Source: CAD feature listing. Evaluate the final solid. Frame: model axes, mm. A direction names the side the tool comes from. Round coordinates to 2 decimals unless told otherwise and drop trailing zeros. Order: outer loops, then holes, each group sorted by start corner. A loop starts at its lowest first (then second) coordinate and runs counter-clockwise, first axis right, second up.
```python
from build123d import *

# Parameters (mm, degrees)
SALIENTE_EXTRUIR1_DEPTH                              = 6.35
REFRENTADO_PARA_TORNILLO_CON_CABEZA_HUEC_D           = 6.7564
REFRENTADO_PARA_TORNILLO_CON_CABEZA_HUEC_CBORE_D     = 11.1125
REFRENTADO_PARA_TORNILLO_CON_CABEZA_HUEC_CBORE_DEPTH = 6.35


with BuildPart() as part:
    # Croquis1 → Saliente-Extruir1 (new, symmetric)
    with BuildSketch(Plane.XY):
        with BuildLine():
            Line((43.5, 63.5), (-43.5, 63.5))
            ThreePointArc((-43.5, 63.5), (-57.642135624, 57.642135624), (-63.5, 43.5))
            Line((-63.5, 43.5), (-63.5, -63.5))
            Line((-63.5, -63.5), (63.5, -63.5))
            Line((63.5, -63.5), (63.5, 43.5))
            ThreePointArc((63.5, 43.5), (57.642135624, 57.642135624), (43.5, 63.5))
        make_face()
    extrude(amount=SALIENTE_EXTRUIR1_DEPTH, both=True)

    # Refrentado para tornillo con cabeza hueca de 1/41 (through all)
    with Locations(Plane(origin=(0, 0, -6.35), x_dir=(-1, 0, 0), z_dir=(0, 0, -1))):
        with Locations((43.85, 34.1), (43.85, 2.1), (-43.85, 2.1), (-43.85, 34.1)):
            CounterBoreHole(REFRENTADO_PARA_TORNILLO_CON_CABEZA_HUEC_D / 2, REFRENTADO_PARA_TORNILLO_CON_CABEZA_HUEC_CBORE_D / 2, REFRENTADO_PARA_TORNILLO_CON_CABEZA_HUEC_CBORE_DEPTH)


solid = part.part
```
1. Line query: line 1 along Y through (x, z) = (-43.85, -3); line 2 along Y through (x, z) = (43.85, 4.5); line 3 along X through (y, z) = (7, -1.5). Output: solid intervals per line, ascending.
2. Pull-direction query (Y, two-part tool) for faces 1 (the face through (-46.531, 32.044, 3.219)), 2 (the face through (-63.5, -9, 0)), 3 (the face through (-57.486, 57.797, 0.089)); classes: released by +Y, released by -Y, zero draft, split by the parting line, or undercut.
3. First-contact query: pin 1 (8 mm diameter, centred on x = -43.85, y = 34.1, fed in from -Z); pin 2 (6.5 mm diameter, centred on x = 43.85, y = 34.1, fed in from +Z); pin 3 (1.5 mm diameter, centred on y = 48.5, z = -4, fed in from -X). Flat tips, straight axial feed; report the tip coordinate or a pass-through.
4. Access query for faces 4 (the face through (1, 63.5, 0)), 5 (the face through (-47.5, 34.2, 0)). Directions: +Z, -Z, +X, -X, +Y, -Y. A direction counts if a zero-diameter tool reaches every point of the face in a straight line with its end or side. Return the directions, or none.
5. Section C-C on x = 45. Return loops of the section in (y, z).
6. Section B-B on y = 2.1. Return loops of the section in (x, z), plus the area to 3 significant figures.
7. Section A-A on z = 2. Return loops of the section in (x, y), plus the area to 3 significant figures.
Result:
1. line 1: y = -63.5 to -3.46, 7.66 to 28.54, 39.66 to 63.5
1. line 2: y = -63.5 to -1.28, 5.48 to 30.72, 37.48 to 63.5
1. line 3: x = -63.5 to -46.47, -41.23 to 41.23, 46.47 to 63.5
2. face 1: undercut
2. face 2: zero draft
2. face 3: released by +Y
3. pin 1: stops at z = 0
3. pin 2: passes through
3. pin 3: stops at x = -63.04
4. face 4: +Z, -Z, +X, -X, +Y
4. face 5: -Z
5. outline: (-63.5, -6.35) - (-3.34, -6.35) - (-3.34, 0) - (-1.08, 0) - (-1.08, 6.35) - (-63.5, 6.35) - close; (5.28, 0) - (7.54, 0) - (7.54, -6.35) - (28.66, -6.35) - (28.66, 0) - (30.92, 0) - (30.92, 6.35) - (5.28, 6.35) - close; (37.28, 0) - (39.54, 0) - (39.54, -6.35) - (63.44, -6.35) - (63.44, 6.35) - (37.28, 6.35) - close
6. outline: (-63.5, -6.35) - (-49.41, -6.35) - (-49.41, 0) - (-47.23, 0) - (-47.23, 6.35) - (-63.5, 6.35) - close; (-40.47, 0) - (-38.29, 0) - (-38.29, -6.35) - (38.29, -6.35) - (38.29, 0) - (40.47, 0) - (40.47, 6.35) - (-40.47, 6.35) - close; (47.23, 0) - (49.41, 0) - (49.41, -6.35) - (63.5, -6.35) - (63.5, 6.35) - (47.23, 6.35) - close
6. area: 1,390 mm2
7. outline: (-63.5, -63.5) - (63.5, -63.5) - (63.5, 43.5) arc R20 ccw to (43.5, 63.5) - (-43.5, 63.5) arc R20 ccw to (-63.5, 43.5) - close; hole circle Ø6.76 at (-43.85, 2.1); hole circle Ø6.76 at (-43.85, 34.1); hole circle Ø6.76 at (43.85, 2.1); hole circle Ø6.76 at (43.85, 34.1)
7. area: 15,800 mm2
